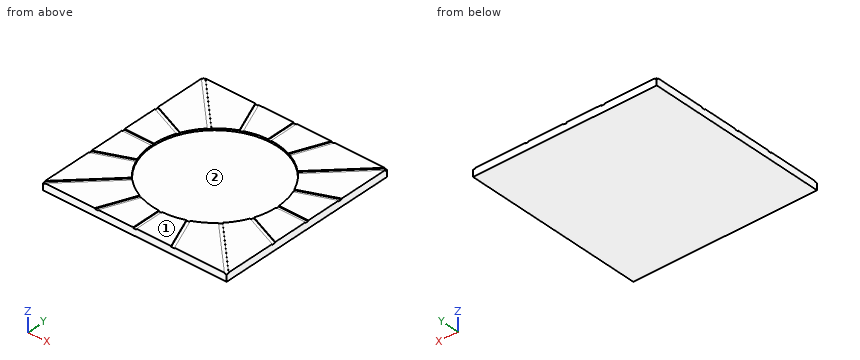
```python
from build123d import *

# Parameters (mm, degrees)
F0_W     = 127
F0_H     = 127
F1_DEPTH = 5.08
F2_W     = 2.19577
F2_H     = 52.046703
F3_DEPTH = 0.508
F4_R     = 43.226331
F5_DEPTH = 1.27


with BuildPart() as f1:
    # F0 (on Top) → F1 (new body)
    with BuildSketch(Plane.XY):
        Rectangle(F0_W, F0_H)
    extrude(amount=F1_DEPTH)

    # F2 (on face) → F3 (cut)
    with BuildSketch(Plane.XY.offset(5.08)):
        Polygon((38.169024, -1.120174), (90.2161, -1.120174), (90.2161, 1.120174), (38.13681, 1.120174), align=None)
        Polygon((-1.096878, -38.1697), (-1.097885, -90.216374), (1.097885, -90.216374), (1.097885, -38.169671), align=None)
        with Locations((0, 64.193022)):
            Rectangle(F2_W, F2_H)
        Polygon((-38.168937, 1.123112), (-90.2161, 1.120174), (-90.2161, -1.120174), (-38.169024, -1.120174), align=None)
        Polygon((27.771347, 26.192397), (64.574188, 62.995238), (62.990023, 64.579402), (26.164404, 27.753783), align=None)
        Polygon((26.204134, -27.77076), (63.005977, -64.574029), (64.558622, -63.021384), (27.756045, -26.218808), align=None)
        Polygon((-63.026599, 64.563836), (-64.579243, 63.011192), (-27.776666, 26.208615), (-26.224022, 27.761259), align=None)
        Polygon((-27.793985, -26.20045), (-64.594809, -63.00543), (-63.010644, -64.589595), (-26.207804, -27.786754), align=None)
        Polygon((35.612549, 13.623586), (83.697778, 33.54114), (82.840434, 35.610951), (34.725444, 15.681069), align=None)
        Polygon((13.513826, -35.632124), (33.430295, -83.717366), (35.458923, -82.877081), (15.541512, -34.792197), align=None)
        Polygon((-33.589701, 83.821042), (-35.618328, 82.980757), (-15.700917, 34.895874), (-13.67229, 35.736159), align=None)
        Polygon((-35.772999, -13.517161), (-83.857183, -33.437463), (-82.999839, -35.507274), (-34.914611, -15.58972), align=None)
        Polygon((34.73032, -15.532565), (82.815549, -35.450119), (83.672893, -33.380308), (35.557903, -13.450427), align=None)
        Polygon((-15.724882, -34.735455), (-35.643213, -82.819926), (-33.614586, -83.660211), (-13.697175, -35.575328), align=None)
        Polygon((35.434038, 83.037912), (33.405411, 83.878197), (13.488, 35.793313), (15.516627, 34.953028), align=None)
        Polygon((-34.938291, 15.753233), (-83.024724, 35.668105), (-83.882068, 33.598294), (-35.796839, 13.68074), align=None)
    extrude(amount=-F3_DEPTH, mode=Mode.SUBTRACT)

    # F4 (on face) → F5 (cut)
    with BuildSketch(Plane.XY.offset(5.08)):
        Circle(F4_R)
    extrude(amount=-F5_DEPTH, mode=Mode.SUBTRACT)


solid = f1.part
```
Part model, mm, in its own coordinate system. Face numbers are marked on the shaded views. Give positions to 0.01 mm unless a question says otherwise; leave off trailing zeros. Loops run counter-clockwise (first coordinate to the right, second up) from the corner with the lowest first, then second, coordinate; pieces in that order, holes last. Notation, with made-up numbers: M 1.5,-29 L 12.5,-29 A18 cw 12.5,-9 Z; hole C 47,-11.5 d9. An arc over 180 degrees is marked long. Return JSON: item names as keys, results as strings.
1) Pull direction X, two halves, no side cores. Call the marked faces 1 and 2: released by +X, released by -X, zero draft, split by the parting line, or undercut.
Calculated:
{"face 1": "zero draft", "face 2": "undercut"}
2) Saw through at A-A, the plane y = -5.5. List the corners of the cut face in (x, z) (3 decimals), then the cut area to 3 significant figures.
Calculated:
{"outline": "M -63.5,0 L 63.5,0 L 63.5,5.08 L 42.875,5.08 L 42.875,3.81 L -42.875,3.81 L -42.875,5.08 L -63.5,5.08 Z", "area": "536 mm2"}
3) Drill centre lines: line 1 (Y direction, x = 0, z = 4.45); line 2 (Y direction, x = -32.5, z = 4.8). Where is each one in solid material? Low to high.
Calculated:
{"line 1": "y = -63.5 to -43.23, 43.23 to 63.5", "line 2": "y = -63.5 to -34.08, -30.91 to -28.5, 28.5 to 30.93, 34.04 to 63.5"}
